from build123d import *

# Parameters (mm, degrees)
SKETCH1_R              = 42.5
BOSS_EXTRUDE1_DEPTH    = 65
SKETCH2_R              = 45.05
CUT_EXTRUDE1_DEPTH     = 23.5
SKETCH3_R              = 44.9925
CUT_EXTRUDE2_DEPTH     = 18
M6_TAPPED_HOLE1_D      = 5.1
M6_TAPPED_HOLE1_DEPTH  = 12
M6_TAPPED_HOLE1_TIP    = 1.532194579
M6_TAPPED_HOLE2_D      = 5.1
M6_TAPPED_HOLE2_DEPTH  = 12
M6_TAPPED_HOLE2_TIP    = 1.532194579
F_12_0MM_DOWEL_HOLE1_D = 13.6


with BuildPart() as part:
    # Sketch1 → Boss-Extrude1 (new body)
    with BuildSketch(Plane.XY):
        with BuildLine():
            Line((6.25, 200.253164472), (6.25, 61.684175442))
            ThreePointArc((6.25, 61.684175442), (0, 62), (-6.25, 61.684175442))
            Line((-6.25, 61.684175442), (-6.25, 200.253164472))
            Line((-6.25, 200.253164472), (-18.25, 200.253164472))
            Line((-18.25, 200.253164472), (-18.25, 59.253164472))
            ThreePointArc((-18.25, 59.253164472), (0, -62), (18.25, 59.253164472))
            Line((18.25, 59.253164472), (18.25, 200.253164472))
            Line((18.25, 200.253164472), (6.25, 200.253164472))
        make_face()
        Circle(SKETCH1_R, mode=Mode.SUBTRACT)
    extrude(amount=BOSS_EXTRUDE1_DEPTH)

    # Sketch2 → Cut-Extrude1 (cut)
    with BuildSketch(Plane.XY.offset(65)):
        Circle(SKETCH2_R)
    extrude(amount=-CUT_EXTRUDE1_DEPTH, mode=Mode.SUBTRACT)

    # Sketch3 → Cut-Extrude2 (cut)
    with BuildSketch(Plane.XY.offset(41.5)):
        Circle(SKETCH3_R)
    extrude(amount=-CUT_EXTRUDE2_DEPTH, mode=Mode.SUBTRACT)

    # M6 Tapped Hole1
    with Locations(Plane.XY.offset(65)):
        with Locations((0, -52.5), (-52.5, 0), (0, 52.5), (52.5, 0)):
            Hole(M6_TAPPED_HOLE1_D / 2, depth=M6_TAPPED_HOLE1_DEPTH)
            with Locations((0, 0, -(M6_TAPPED_HOLE1_DEPTH + M6_TAPPED_HOLE1_TIP / 2))):  # 118° drill point
                Cone(0, M6_TAPPED_HOLE1_D / 2, M6_TAPPED_HOLE1_TIP, mode=Mode.SUBTRACT)

    # M6 Tapped Hole2
    with Locations(Plane(origin=(0, 0, 0), x_dir=(-1, 0, 0), z_dir=(0, 0, -1))):
        with Locations((-52.5, 0), (0, 52.5), (52.5, 0), (0, -52.5)):
            Hole(M6_TAPPED_HOLE2_D / 2, depth=M6_TAPPED_HOLE2_DEPTH)
            with Locations((0, 0, -(M6_TAPPED_HOLE2_DEPTH + M6_TAPPED_HOLE2_TIP / 2))):  # 118° drill point
                Cone(0, M6_TAPPED_HOLE2_D / 2, M6_TAPPED_HOLE2_TIP, mode=Mode.SUBTRACT)

    # Ø12.0mm Dowel Hole1 (through all)
    with Locations(Plane(origin=(18.25, 0, 0), x_dir=(0, 0, -1), z_dir=(1, 0, 0))):
        with Locations((-50, 175.253164472), (-15, 175.253164472), (-15, 115.253164472), (-50, 115.253164472)):
            Hole(F_12_0MM_DOWEL_HOLE1_D / 2)


solid = part.part
Geometry check sheet. Reference: the model listing, model coordinates, mm. A direction names the side the tool comes from. Round coordinates to 2 decimals unless told otherwise and drop trailing zeros. Write each loop counter-clockwise with the first axis right and the second up, starting at its lowest first coordinate (ties: lowest second). Pieces come first, ordered by that corner, then holes. Notation, with made-up numbers: (48, 9.5) -> (64, 9.5) arc R19 cw to (64, 25.5) -> close; hole circle Ø1 at (-19.75, 35.5). An arc over 180 degrees is marked (long way). One line per item, written item: value. Start each with the question number.
(1) Cross-section at B-B, the plane y = 132. Record the cut outline in (x, z).
(2) Scan lines: line 1 (X direction, y = 0, z = 5.25); line 2 (X direction, y = 187, z = 19.5); line 3 (X direction, y = 0, z = 17.25). Record each from-to range of solid material in increasing order. Write a range as [from, to].
(3) Cross-section at D-D, the plane z = 48.5. Record the cut outline in (x, y), and give its area (3 significant figures).
(4) Access from +Z, -Z, +X, -X, +Y, -Y to the whole of each face (thin tool, end or side, straight path). Record for faces 4 (the flat face through (12, 200.253, 32)), 5 (the flat face through (6.25, 132, 32)), 6 (the cylindrical face through (0.33, 55.03, 58.92)), 7 (the cylindrical face through (-0.33, -49.97, 6.08)), 8 (the cylindrical face through (12.166, 180.987, 53.656)).
(5) Draft check along Y on faces 1 (the conical face through (-0.096, 52.068, 51.734)), 2 (the flat face through (-12, 200.253, 32)), 3 (the flat face through (4, 50, 65)). Enter one of: +Y half, -Y half, draft (parallel to the pull), parting line (faces both ways), or undercut.
(6) Cross-section at C-C, the plane x = -11. Record the cut outline in (y, z).
(7) Go/stop test with flat-tipped pins: pin 1 Ø11 at (y, z) = (175.25, 50) entering from -X; pin 2 Ø4 at (x, y) = (0, -52.5) entering from +Z; pin 3 Ø4.5 at (x, y) = (52.5, 0) entering from +Z; pin 4 Ø12 at (y, z) = (139, 34.5) entering from +X. Record where each tip stops, or that it passes through.
Answer:
1. outline: (-18.25, 0) -> (-6.25, 0) -> (-6.25, 65) -> (-18.25, 65) -> close; (6.25, 0) -> (18.25, 0) -> (18.25, 65) -> (6.25, 65) -> close
2. line 1: [-62, -55.05], [-49.95, -42.5], [42.5, 49.95], [55.05, 62]
2. line 2: [-18.25, -6.25], [6.25, 18.25]
2. line 3: [-62, -42.5], [42.5, 62]
3. outline: (-18.25, 59.25) arc R62 ccw (long way) to (18.25, 59.25) -> (18.25, 108.62) -> (6.25, 108.62) -> (6.25, 61.68) arc R62 ccw to (-6.25, 61.68) -> (-6.25, 108.62) -> (-18.25, 108.62) -> close; (-18.25, 121.89) -> (-6.25, 121.89) -> (-6.25, 168.62) -> (-18.25, 168.62) -> close; (-18.25, 181.89) -> (-6.25, 181.89) -> (-6.25, 200.25) -> (-18.25, 200.25) -> close; (6.25, 121.89) -> (18.25, 121.89) -> (18.25, 168.62) -> (6.25, 168.62) -> close; (6.25, 181.89) -> (18.25, 181.89) -> (18.25, 200.25) -> (6.25, 200.25) -> close; hole circle Ø90.1 at (0, 0)
3. area: 8,410 mm²
4. face 4: +Z, -Z, +X, -X, +Y
4. face 5: +Z, -Z, +Y
4. face 6: +Z
4. face 7: -Z
4. face 8: +X, -X
5. face 1: undercut
5. face 2: +Y half
5. face 3: draft
6. outline: (-61.02, 0) -> (-41.05, 0) -> (-41.05, 23.5) -> (-43.63, 23.5) -> (-43.63, 41.5) -> (-43.69, 41.5) -> (-43.69, 65) -> (-61.02, 65) -> close; (41.05, 0) -> (200.25, 0) -> (200.25, 65) -> (43.69, 65) -> (43.69, 41.5) -> (43.63, 41.5) -> (43.63, 23.5) -> (41.05, 23.5) -> close; hole circle Ø13.6 at (115.25, 15); hole circle Ø13.6 at (115.25, 50); hole circle Ø13.6 at (175.25, 15); hole circle Ø13.6 at (175.25, 50)
7. pin 1: through
7. pin 2: z = 52.67
7. pin 3: z = 52.82
7. pin 4: x = 18.25
